```python
from build123d import *

# Parameters (mm, degrees)
F1_DEPTH = 12.7
F2_DEPTH = 3.048


with BuildPart() as f1:
    # F0 (on Front) → F1 (new body)
    with BuildSketch(Plane.XZ):
        with BuildLine():
            Line((0, 51.2216350224), (0, 53.6040686))
            ThreePointArc((0, 53.6040686), (-7.1342213589, 56.8180852692), (-9.4538482046, 64.2911267413))
            Line((-9.4538482046, 64.2911267413), (-15.3375121761, 16.4249623056))
            ThreePointArc((-15.3375121761, 16.4249623056), (-9.6693668982, 24.9195002363), (0, 28.2040686))
            Line((0, 28.2040686), (0, 46.4869021777))
            ThreePointArc((0, 46.4869021777), (-7.5126241699, 48.8542686), (0, 51.2216350224))
        make_face()
        with BuildLine():
            ThreePointArc((9.525, 63.1290686), (6.7351920908, 56.3938765092), (0, 53.6040686))
            Line((0, 53.6040686), (0, 51.2216350224))
            ThreePointArc((0, 51.2216350224), (0.5550872912, 50.0953307458), (0.7460008182, 48.8542686))
            ThreePointArc((0.7460008182, 48.8542686), (0.5550872912, 47.6132064543), (0, 46.4869021777))
            Line((0, 46.4869021777), (0, 28.2040686))
            ThreePointArc((0, 28.2040686), (9.6519445425, 24.9328613447), (15.3261239176, 16.4673714724))
            Line((15.3261239176, 16.4673714724), (9.525, 63.1290686))
        make_face()
        with BuildLine():
            ThreePointArc((-9.4538482046, 64.2911267413), (-7.1342213589, 56.8180852692), (0, 53.6040686))
            ThreePointArc((0, 53.6040686), (6.7351920908, 56.3938765092), (9.525, 63.1290686))
            ThreePointArc((9.525, 63.1290686), (0.5821171922, 72.6362640106), (-9.4538482046, 64.2911267413))
        make_face()
        with BuildLine():
            ThreePointArc((3.175, 63.1290686), (2.2450640303, 60.8840045698), (0, 59.9540686))
            ThreePointArc((0, 59.9540686), (-2.2450640303, 65.3741326303), (3.175, 63.1290686))
        make_face(mode=Mode.SUBTRACT)
        with BuildLine():
            Line((15.8728781179, 12.0695204249), (15.3261239176, 16.4673714724))
            ThreePointArc((15.3261239176, 16.4673714724), (9.6519445425, 24.9328613447), (0, 28.2040686))
            Line((0, 28.2040686), (0, 16.9626167222))
            ThreePointArc((0, 16.9626167222), (3.2764132981, 15.6054818982), (4.6335481221, 12.3290686))
            ThreePointArc((4.6335481221, 12.3290686), (3.2764132981, 9.0526553019), (0, 7.6955204779))
            Line((0, 7.6955204779), (0, -3.5459314))
            ThreePointArc((0, -3.5459314), (10.1482027408, 0.1213003301), (15.6077993594, 9.4286851503))
            Line((15.6077993594, 9.4286851503), (15.8728781179, 12.0695204249))
        make_face()
        with BuildLine():
            ThreePointArc((0, 28.2040686), (-9.6693668982, 24.9195002363), (-15.3375121761, 16.4249623056))
            Line((-15.3375121761, 16.4249623056), (-15.8728782216, 12.0695267661))
            Line((-15.8728782216, 12.0695267661), (-15.6120639675, 9.4517289128))
            ThreePointArc((-15.6120639675, 9.4517289128), (-10.1572106768, 0.1287941659), (0, -3.5459314))
            Line((0, -3.5459314), (0, 7.6955204779))
            ThreePointArc((0, 7.6955204779), (-4.6335481221, 12.3290686), (0, 16.9626167222))
            Line((0, 16.9626167222), (0, 28.2040686))
        make_face()
        with BuildLine():
            ThreePointArc((0, -3.5459314), (-10.1572106768, 0.1287941659), (-15.6120639675, 9.4517289128))
            Line((-15.6120639675, 9.4517289128), (-9.4780747266, -52.1152430422))
            ThreePointArc((-9.4780747266, -52.1152430422), (-7.0611682246, -44.7783162619), (0, -41.6459314))
            Line((0, -41.6459314), (0, -3.5459314))
        make_face()
        with BuildLine():
            ThreePointArc((0, -41.6459314), (-7.0611682246, -44.7783162619), (-9.4780747266, -52.1152430422))
            ThreePointArc((-9.4780747266, -52.1152430422), (-6.3926151381, -58.2320996246), (0, -60.6959314))
            Line((0, -60.6959314), (0.6773435479, -60.6718171859))
            ThreePointArc((0.6773435479, -60.6718171859), (6.9705567315, -57.6622304882), (9.525, -51.1709314))
            Line((9.525, -51.1709314), (3.175, -51.1709314))
            ThreePointArc((3.175, -51.1709314), (-2.2450640303, -53.4159954302), (0, -47.9959314))
            Line((0, -47.9959314), (0, -41.6459314))
        make_face()
        with BuildLine():
            ThreePointArc((9.525, -51.1709314), (6.7351920908, -44.4357393092), (0, -41.6459314))
            Line((0, -41.6459314), (0, -47.9959314))
            ThreePointArc((0, -47.9959314), (2.2450640303, -48.9258673697), (3.175, -51.1709314))
            Line((3.175, -51.1709314), (9.525, -51.1709314))
        make_face()
        with BuildLine():
            Line((11.290697226, -33.5802517612), (15.6077993594, 9.4286851503))
            ThreePointArc((15.6077993594, 9.4286851503), (10.1482027408, 0.1213003301), (0, -3.5459314))
            Line((0, -3.5459314), (0, -41.6459314))
            ThreePointArc((0, -41.6459314), (6.7351920908, -44.4357393092), (9.525, -51.1709314))
            Line((9.525, -51.1709314), (36.5125, -51.1709314))
            ThreePointArc((36.5125, -51.1709314), (38.9380895153, -45.459298616), (44.7324052746, -43.2384567854))
            Line((44.7324052746, -43.2384567854), (18.9182890587, -42.3194443799))
            ThreePointArc((18.9182890587, -42.3194443799), (13.2114936015, -39.60206338), (11.290697226, -33.5802517612))
        make_face()
        with BuildLine():
            Line((36.5125, -51.1709314), (9.525, -51.1709314))
            ThreePointArc((9.525, -51.1709314), (6.9705567315, -57.6622304882), (0.6773435479, -60.6718171859))
            Line((0.6773435479, -60.6718171859), (44.7324052746, -59.1034060145))
            ThreePointArc((44.7324052746, -59.1034060145), (38.9380895153, -56.8825641839), (36.5125, -51.1709314))
        make_face()
        with BuildLine():
            ThreePointArc((52.3875, -51.1709314), (50.1616327839, -45.6590209152), (44.7324052746, -43.2384567854))
            ThreePointArc((44.7324052746, -43.2384567854), (38.9380895153, -45.459298616), (36.5125, -51.1709314))
            ThreePointArc((36.5125, -51.1709314), (38.9380895153, -56.8825641839), (44.7324052746, -59.1034060145))
            ThreePointArc((44.7324052746, -59.1034060145), (50.1616327839, -56.6828418847), (52.3875, -51.1709314))
        make_face()
        with BuildLine():
            ThreePointArc((48.30468059, -51.1709314), (44.45, -55.02561199), (40.59531941, -51.1709314))
            ThreePointArc((40.59531941, -51.1709314), (44.45, -47.3162508099), (48.30468059, -51.1709314))
        make_face(mode=Mode.SUBTRACT)
    extrude(amount=F1_DEPTH)

    # F0 (on Front) → F2 (join)
    with BuildSketch(Plane.XZ):
        with BuildLine():
            ThreePointArc((9.525, -51.1709314), (6.7351920908, -44.4357393092), (0, -41.6459314))
            Line((0, -41.6459314), (0, -47.9959314))
            ThreePointArc((0, -47.9959314), (2.2450640303, -48.9258673697), (3.175, -51.1709314))
            Line((3.175, -51.1709314), (9.525, -51.1709314))
        make_face()
    extrude(amount=F2_DEPTH)


solid = f1.part
```
Work out the finished part from the listing and answer in its coordinate system (mm). A direction names the side the tool comes from. Round coordinates to 2 decimals unless told otherwise and drop trailing zeros. Write each loop counter-clockwise with the first axis right and the second up, starting at its lowest first coordinate (ties: lowest second). Pieces come first, ordered by that corner, then holes.
1) A cutting plane is placed at C-C on x = 31.5. Determine the outline of the cut face in (y, z), and give its area (3 significant figures).
2) Consider probe 1 along Z at (x, y) = (-1.5, -7.5); probe 2 along Z at (x, y) = (-1, -7.75); probe 3 along Z at (x, y) = (38, -1.75). Determine where each line is inside the solid, lowest interval first.
3) A cutting plane is placed at D-D on z = -12. Determine the outline of the cut face in (x, y).
4) Flat-ended cylindrical pins translate along their axes: P1, Ø4, axis at y = -7.5, z = -4, coming from the -X side; P2, Ø3, axis at x = 9.5, y = -6, coming from the +Z side; P3, Ø3, axis at x = 11, y = -6, coming from the -Z side. Find the tip coordinate at first contact, or state that the pin passes through.
5) A cutting plane is placed at B-B on y = -8. Give the number of separate pieces and of enclosed holes in the cut face, and give its area (3 significant figures).
6) Which of the six approach directions +Z, -Z, +X, -X, +Y, -Y give full straight-line access (tool end or side, diameter ignored) to faces 1 (the face through (3, 0, -8)), 2 (the face through (13.3, -6.3, -39.7))?
7) A cutting plane is placed at A-A on z = 14.5. Determine the outline of the cut face in (x, y).
Entries:
1. outline: (-12.7, -59.57) - (0, -59.57) - (0, -42.77) - (-12.7, -42.77) - close
1. area: 213 mm2
2. probe 1: z = -60.58 to -53.97, -48.37 to 7.95, 16.71 to 45.18, 52.53 to 60.33, 65.93 to 72.54
2. probe 2: z = -60.64 to -54.18, -48.16 to 7.8, 16.85 to 45.48, 52.23 to 60.12, 66.14 to 72.6
2. probe 3: z = -59.34 to -43
3. outline: (-13.47, -12.7) - (13.46, -12.7) - (13.46, 0) - (-13.47, 0) - close
4. P1: stops at x = -14.47
4. P2: stops at z = 68.3
4. P3: stops at z = -60.36
5. separate pieces: 1
5. enclosed holes: 5
5. area: 3,690 mm2
6. face 1: +Z, -Z, +X, -X, +Y
6. face 2: +X, +Y, -Y
7. outline: (-15.57, -12.7) - (-4.09, -12.7) - (-4.09, 0) - (-15.57, 0) - close; (4.09, -12.7) - (15.57, -12.7) - (15.57, 0) - (4.09, 0) - close
